Model file for the job. Use its own axes, mm. A direction names the side the tool comes from. Coordinates: 2 decimals unless noted, no trailing zeros. Write each loop counter-clockwise with the first axis right and the second up, starting at its lowest first coordinate (ties: lowest second). Pieces come first, ordered by that corner, then holes. Notation, with made-up numbers: M 64,-18.5 L 98,-18.5 A6 ccw 98,-12.5 Z; hole C 87,66 d3. An arc over 180 degrees is marked long. Use CSV: the item, a comma, the result in double quotes. Start each with the question number.
Autodesk Inventor part; units mm, degrees
ref_plane "YZ Plane" through (0, 0, 0) normal (1, 0, 0) x (0, 1, 0)
ref_plane "XZ Plane" through (0, 0, 0) normal (0, 1, 0) x (-1, 0, 0)
ref_plane "XY Plane" through (0, 0, 0) normal (0, 0, 1) x (1, 0, 0)
sketch "Esquisse1" plane through (0, 0, 0) normal (0, 0, 1) x (1, 0, 0)
  line L0 (-20, -20) -> (20, -20)
  line L1 (20, -20) -> (20, 20)
  line L2 (20, 20) -> (-20, 20)
  line L3 (-20, 20) -> (-20, -20)
  line L4 (-20, -20) -> (20, 20) construction
  line L5 (20, -20) -> (-20, 20) construction
  point P0 (0, 0)
  dimension "d0" = 40
  dimension "d1" = 40
extrude "Extrusion1" add sketch "Esquisse1" along normal blind 4.75
sketch "Esquisse2" plane through (0, 0, 0) normal (0, 0, -1) x (-1, 0, 0)
  circle A0 centre (0, 0) radius 18
  dimension "d4" = 36
extrude "Extrusion2" add sketch "Esquisse2" along normal blind 22.5
sketch "Esquisse3" plane through (0, 0, -22.5) normal (0, 0, -1) x (-1, 0, 0)
  circle A0 centre (0, 0) radius 11
  dimension "d7" = 22
extrude "Extrusion3" add sketch "Esquisse3" along normal blind 2
sketch "Esquisse4" plane through (0, 0, -24.5) normal (0, 0, -1) x (-1, 0, 0)
  circle A0 centre (0, 0) radius 4
  dimension "d10" = 8
extrude "Extrusion4" add sketch "Esquisse4" along normal blind 18
sketch "Esquisse5" plane through (0, 0, -22.5) normal (0, 0, -1) x (-1, 0, 0)
  line L0 (2.75, 14) -> (2.75, 20)
  line L1 (2.75, 20) -> (-2.75, 20)
  line L2 (-2.75, 20) -> (-2.75, 14)
  arc A0 (-2.75, 14) -> (2.75, 14) centre (0, 14) ccw
  line L3 (-5.8727, 11.25) -> (6.9121, 11.25) construction
  line L4 (-20, 20) -> (20, 20) construction
  point P0 (0, 0)
  dimension "d13" = 5.5
  dimension "d14" = 11.25
extrude "Extrusion5" cut sketch "Esquisse5" against normal blind 3.85
pattern_circular "Réseau circulaire1" count 4 over 360 about axis through (0, 0, 0) along (0, 0, -1) of "Extrusion5"
sketch "Esquisse6" plane through (0, 0, -22.5) normal (0, 0, -1) x (-1, 0, 0)
  circle A0 centre (0, 0) radius 14 construction
  circle A1 centre (0, 0) radius 11 construction
  line L0 (0, 0) -> (-20.9292, 20.9292) construction
  line L1 (28, 0) -> (-28, 0) construction
  point P0 (-9.8995, 9.8995)
  dimension "d20" = 28
  dimension "d21" = 45
hole "Perçage1" at (9.8995, 9.8995, -22.5) direction (0, 0, 1) diameter 2.459 depth 8.8 tip angle 118
pattern_circular "Réseau circulaire2" count 4 over 360 about axis through (0, 0, 0) along (0, 0, -1) of "Perçage1"
sketch "Esquisse7" plane through (0, 0, 0) normal (0, 0, -1) x (-1, 0, 0)
  point P0 (0, 0)
  point P1 (15.5, 15.5)
  point P2 (15.5, -15.5)
  point P3 (-15.5, -15.5)
  point P4 (-15.5, 15.5)
  dimension "d32" = 31
  dimension "d33" = 31
  dimension "d34" = 15.5
  dimension "d35" = 15.5
hole "Perçage2" at (-15.5, 15.5, 0) at (-15.5, -15.5, 0) at (15.5, -15.5, 0) at (15.5, 15.5, 0) direction (0, 0, 1) diameter 3.5 end through all counterbore diameter 6 counterbore depth 3
chamfer "Chanfrein1" distance 4 angle 45 4 edges at (-20, -20, 2.375) (20, -20, 2.375) (20, 20, 2.375) (-20, 20, 2.375)
fillet "Congé1" radius 2 8 edges at (-16, -20, 2.375) (16, -20, 2.375) (20, -16, 2.375) (20, 16, 2.375) (16, 20, 2.375) (-16, 20, 2.375) (-20, 16, 2.375) (-20, -16, 2.375)
properties part number "Reducteur" material "----------"
1) Wall check: L1, parallel to Y at x = -10.5, z = -21; L2, parallel to X at y = -15, z = 4; L3, parallel to Y at x = 15, z = 2. Give the ranges that are in metal, low to high. Write a range as [from, to].
2) Drop flat-ended pins along their axis: P1, Ø3, axis at y = 9.5, z = -1, coming from the +X side; P2, Ø1.5, axis at y = -2, z = -19, coming from the +X side; P3, Ø1.8, axis at x = -14, y = -16.5, coming from the -Z side; P4, Ø3, axis at x = 16.5, z = -20.5, coming from the +Y side. Give the stop position or say it passes through.
3) Band-saw the part on B-B on z = -32.5. List the corners of the cut face in (x, y).
4) Band-saw the part on A-A on y = 0. List the corners of the cut face in (x, z), then the cut area to 3 significant figures.
5) Band-saw the part on C-C on x = -2. List the corners of the cut face in (y, z).
6) Band-saw the part on D-D on y = -6. List the corners of the cut face in (x, z), then the cut area to 3 significant figures.
7) Two-plate mould, pull along X, no slides. Class faces 5 (the face through (0.06, 11.25, -20.6)), 6 (the face through (16, -2.75, -21)), 7 (the face through (11.25, -0.06, -20.6)), 8 (the face through (-18, 18, 2)): pulls with the +X half, pulls with the -X half, needs draft (parallel to the pull), parting line crosses it, or undercut.
8) Tool access for faces 1 (the face through (16, 2.75, -21)), 2 (the face through (-0.06, -11.25, -20.6)), 3 (the face through (17, -14, 3)), 4 (the face through (-2.75, 16, -21)): list every direction of +Z, -Z, +X, -X, +Y, -Y with a clear straight run to the whole face (end or side of a thin tool).
Findings below:
1,L1,"y = [-14.62, -10.97], [-8.83, 8.83], [10.97, 14.62]"
1,L2,"x = [-20, -17.18], [-13.82, 13.82], [17.18, 20]"
1,L3,"y = [-20, -18.46], [-12.54, 12.54], [18.46, 20]"
2,P1,"stops at x = 20"
2,P2,"stops at x = 17.95"
2,P3,"stops at z = 3"
2,P4,"stops at y = 9.95"
3,outline,"C 0,0 d8"
4,outline,"M -20,0 L -18,0 L -18,-18.65 L -11.25,-18.65 L -11.25,-22.5 L -11,-22.5 L -11,-24.5 L -4,-24.5 L -4,-42.5 L 4,-42.5 L 4,-24.5 L 11,-24.5 L 11,-22.5 L 11.25,-22.5 L 11.25,-18.65 L 18,-18.65 L 18,0 L 20,0 L 20,4.75 L -20,4.75 Z"
4,area,"1,140 mm2"
5,outline,"M -20,0 L -17.89,0 L -17.89,-18.65 L -12.11,-18.65 L -12.11,-22.5 L -10.82,-22.5 L -10.82,-24.5 L -3.46,-24.5 L -3.46,-42.5 L 3.46,-42.5 L 3.46,-24.5 L 10.82,-24.5 L 10.82,-22.5 L 12.11,-22.5 L 12.11,-18.65 L 17.89,-18.65 L 17.89,0 L 20,0 L 20,4.75 L -20,4.75 Z"
6,outline,"M -20,0 L -16.97,0 L -16.97,-22.5 L -9.22,-22.5 L -9.22,-24.5 L 9.22,-24.5 L 9.22,-22.5 L 16.97,-22.5 L 16.97,0 L 20,0 L 20,4.75 L -20,4.75 Z"
6,area,"991 mm2"
7,face 5,"undercut"
7,face 6,"needs draft"
7,face 7,"pulls with the +X half"
7,face 8,"pulls with the -X half"
8,face 1,"-Z, +X"
8,face 2,"-Z, -Y"
8,face 3,"-Z"
8,face 4,"-Z, +Y"
